Could you check a few things on this model? Use its own coordinates, in mm. A direction names the side the tool comes from. Round coordinates to 2 decimals unless told otherwise and drop trailing zeros. Loops run counter-clockwise (first coordinate to the right, second up) from the corner with the lowest first, then second, coordinate; pieces in that order, holes last. Notation, with made-up numbers: (-23, 54) -> (-9, 54) arc R25 cw to (-9, 74) -> close; hole circle Ø3 at (84, 8.5). An arc over 180 degrees is marked (long way). One line per item, written item: value.
from build123d import *

# Parameters (mm, degrees)
CROQUIS1_R              = 26
CROQUIS1_R_2            = 12.5
SALIENTE_EXTRUIR1_DEPTH = 3


with BuildPart() as part:
    # Croquis1 → Saliente-Extruir1 (new body)
    with BuildSketch(Plane(origin=(0, 0, 0), x_dir=(0, 0, -1), z_dir=(1, 0, 0))):
        Polygon((-23, 82), (23, 82), (23, 85), (47.5, 85), (47.5, 23), (44.5, 23), (44.5, -23), (47.5, -23), (47.5, -85), (23, -85), (23, -82), (-23, -82), (-23, -85), (-47.5, -85), (-47.5, -23), (-44.5, -23), (-44.5, 23), (-47.5, 23), (-47.5, 85), (-23, 85), align=None)
        with Locations((0, 31)):
            Circle(CROQUIS1_R, mode=Mode.SUBTRACT)
        with Locations((0, -49.5)):
            Circle(CROQUIS1_R_2, mode=Mode.SUBTRACT)
    extrude(amount=SALIENTE_EXTRUIR1_DEPTH)


solid = part.part
(1) If we section it at A-A, the plane z = 0: Please give me the cut outline in (x, y).
Recorded:
outline: (0, -82) -> (3, -82) -> (3, -62) -> (0, -62) -> close; (0, -37) -> (3, -37) -> (3, 5) -> (0, 5) -> close; (0, 57) -> (3, 57) -> (3, 82) -> (0, 82) -> close
(2) If we section it at B-B, the plane y = -49.5: Please give me the cut outline in (x, z).
Recorded:
outline: (0, -47.5) -> (3, -47.5) -> (3, -12.5) -> (0, -12.5) -> close; (0, 12.5) -> (3, 12.5) -> (3, 47.5) -> (0, 47.5) -> close
(3) Thinking about a two-plate mould opening in Y: for faces 1 (the face through (1, -84, -23)), 2 (the face through (1, -85, 35)), 3 (the face through (1, 23, 46)), which applies, released by +Y, released by -Y, zero draft, split by the parting line, or undercut?
Recorded:
face 1: zero draft
face 2: released by -Y
face 3: undercut
(4) I'm going to push flat-ended pins straight in: pin 1 Ø1.5 at (x, y) = (2, -11) entering from +Z; pin 2 Ø1.5 at (x, y) = (2, 9.5) entering from -Z; pin 3 Ø1.5 at (x, z) = (1.5, 9.5) entering from +Y. Where does each tip first touch, or does it pass through?
Recorded:
pin 1: z = 44.5
pin 2: z = -44.5
pin 3: y = 82
(5) If we section it at D-D, the plane z = 21: Please give me the cut outline in (x, y), then the cut area to 3 significant figures.
Recorded:
outline: (0, -82) -> (3, -82) -> (3, 15.67) -> (0, 15.67) -> close; (0, 46.33) -> (3, 46.33) -> (3, 82) -> (0, 82) -> close
area: 400 mm²
(6) If we section it at C-C, the plane x = 1.4: Please give me the cut outline in (y, z), then the cut area to 3 significant figures.
Recorded:
outline: (-85, -47.5) -> (-23, -47.5) -> (-23, -44.5) -> (23, -44.5) -> (23, -47.5) -> (85, -47.5) -> (85, -23) -> (82, -23) -> (82, 23) -> (85, 23) -> (85, 47.5) -> (23, 47.5) -> (23, 44.5) -> (-23, 44.5) -> (-23, 47.5) -> (-85, 47.5) -> (-85, 23) -> (-82, 23) -> (-82, -23) -> (-85, -23) -> close; hole circle Ø25 at (-49.5, 0); hole circle Ø52 at (31, 0)
area: 13,000 mm²
(7) For faces 4 (the face through (1, -23, -46)), 5 (the face through (1, -82, 0)), 6 (the face through (1, 0, 44.5)), 7 (the face through (1, 82, 0)), which set-ups out of +Z, -Z, +X, -X, +Y, -Y let a thin tool reach every point of the face, with its end or its side?
Recorded:
face 4: -Z, +X, -X
face 5: +X, -X, -Y
face 6: +Z, +X, -X
face 7: +X, -X, +Y
(8) If I drill on L1, parallel to Y at x = 1.7, z = 0; L2, parallel to Y at x = 2.55, z = 2; L3, parallel to Z at x = 0.85, y = -49, over which ranges is the centre line in solid material (lowest first)?
Recorded:
L1: -82 to -62, -37 to 5, 57 to 82
L2: -82 to -61.84, -37.16 to 5.08, 56.92 to 82
L3: -47.5 to -12.49, 12.49 to 47.5
